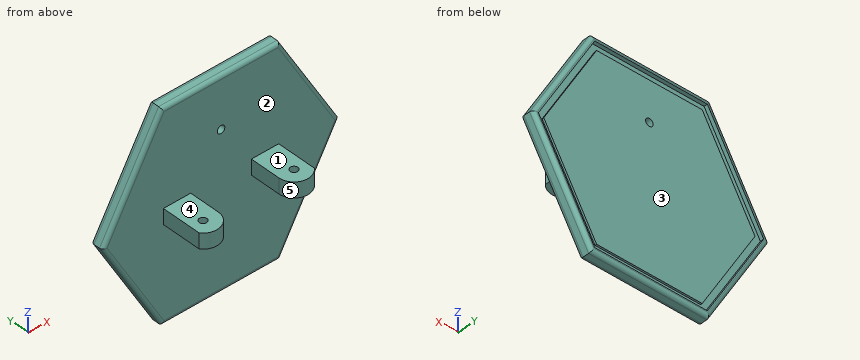
Autodesk Inventor part; units mm, degrees
ref_plane "YZ Plane" through (0, 0, 0) normal (1, 0, 0) x (0, 1, 0)
ref_plane "XZ Plane" through (0, 0, 0) normal (0, 1, 0) x (-1, 0, 0)
ref_plane "XY Plane" through (0, 0, 0) normal (0, 0, 1) x (1, 0, 0)
sketch "스케치1" plane through (0, 0, 0) normal (0, 1, 0) x (-1, 0, 0)
  line L0 (17.6385, -30.5508) -> (-17.6385, -30.5508)
  line L1 (-17.6385, -30.5508) -> (-35.277, 0)
  line L2 (-35.277, 0) -> (-17.6385, 30.5508)
  line L3 (-17.6385, 30.5508) -> (17.6385, 30.5508)
  line L4 (17.6385, 30.5508) -> (35.277, 0)
  line L5 (35.277, 0) -> (17.6385, -30.5508)
  line L6 (19.486, -33.7508) -> (-19.486, -33.7508)
  line L7 (-19.486, -33.7508) -> (-38.972, 0)
  line L8 (-38.972, 0) -> (-19.486, 33.7508)
  line L9 (-19.486, 33.7508) -> (19.486, 33.7508)
  line L10 (19.486, 33.7508) -> (38.972, 0)
  line L11 (38.972, 0) -> (19.486, -33.7508)
  point P0 (0, 0)
  point P1 (0, 0)
  point P2 (0, 0)
  dimension "d0" = 70.554
  dimension "d1" = 3.2
extrude "돌출1" add sketch "스케치1" along normal blind 4.4 contours L0 L1 L2 L3 L4 L5 | L6 L7 L8 L9 L10 L11
sketch "스케치2" plane through (0, 4.4, 0) normal (0, 1, 0) x (1, 0, 0)
  line L0 (-18.5623, 32.1508) -> (18.5623, 32.1508)
  line L1 (18.5623, 32.1508) -> (37.1245, 0)
  line L2 (37.1245, 0) -> (18.5623, -32.1508)
  line L3 (18.5623, -32.1508) -> (-18.5623, -32.1508)
  line L4 (-18.5623, -32.1508) -> (-37.1245, 0)
  line L5 (-37.1245, 0) -> (-18.5623, 32.1508)
  line L6 (-19.486, 33.7508) -> (-38.972, 0)
  point P0 (0, 0)
  point P1 (0, 0)
  dimension "d4" = 1.6
extrude "돌출2" cut sketch "스케치2" against normal blind 1.2
sketch "스케치3" plane through (0, 3.2, 0) normal (0, 1, 0) x (1, 0, 0)
  line L0 (17.4076, -30.1508) -> (-17.4076, -30.1508)
  line L1 (-17.4076, -30.1508) -> (-34.8151, 0)
  line L2 (-34.8151, 0) -> (-17.4076, 30.1508)
  line L3 (-17.4076, 30.1508) -> (17.4076, 30.1508)
  line L4 (17.4076, 30.1508) -> (34.8151, 0)
  line L5 (34.8151, 0) -> (17.4076, -30.1508)
  line L6 (-18.5623, 32.1508) -> (18.5623, 32.1508)
  point P0 (0, 0)
  point P1 (0, 0)
  dimension "d7" = 2
extrude "돌출3" add sketch "스케치3" along normal blind 0.6
fillet "모깎기1" radius 1.2 12 edges at (0, 4.4, -33.7508) (0, 0, -33.7508) (-29.229, 4.4, -16.8754) (-29.229, 0, -16.8754) (-29.229, 4.4, 16.8754) (-29.229, 0, 16.8754) (0, 0, 33.7508) (0, 4.4, 33.7508) (29.229, 0, 16.8754) (29.229, 4.4, 16.8754) (29.229, 4.4, -16.8754) (29.229, 0, -16.8754)
sketch "스케치6" plane through (0, 0, 0) normal (0, -1, 0) x (1, 0, 0)
  line L0 (-20, -2.5) -> (-10, -2.5)
  line L1 (-10, -2.5) -> (-10, 2.5)
  line L2 (-10, 2.5) -> (-20, 2.5)
  line L3 (-20, 2.5) -> (-20, -2.5)
  line L4 (-20, -2.5) -> (-10, 2.5) construction
  line L5 (-10, -2.5) -> (-20, 2.5) construction
  line L6 (10, -2.5) -> (20, -2.5)
  line L7 (20, -2.5) -> (20, 2.5)
  line L8 (20, 2.5) -> (10, 2.5)
  line L9 (10, 2.5) -> (10, -2.5)
  line L10 (10, -2.5) -> (20, 2.5) construction
  line L11 (20, -2.5) -> (10, 2.5) construction
  point P0 (0, 0)
  point P1 (-15, 0)
  point P2 (15, 0)
  point P3 (-10, 0)
  point P4 (10, 0)
  dimension "d27" = 10
  dimension "d28" = 5
  dimension "d29" = 10
  dimension "d30" = 5
  dimension "d31" = 20
  dimension "d32" = 10
extrude "돌출6" add sketch "스케치6" along normal blind 10
sketch "스케치7" plane through (-10, 0, -2.5) normal (0, 0, -1) x (-1, 0, 0)
  line L0 (10, -10) -> (0, -10)
  circle A0 centre (5, -10) radius 5
  line L1 (-30, -10) -> (-20, -10)
  circle A1 centre (-25, -10) radius 5
  point P0 (-10, 0)
extrude "돌출7" add sketch "스케치7" against normal blind 5
sketch "스케치8" plane through (-10, 0, -2.5) normal (0, 0, -1) x (-1, 0, 0)
  arc A0 (0, -10) -> (10, -10) centre (5, -10) ccw
  circle A1 centre (5, -10) radius 1.25
  arc A2 (-30, -10) -> (-20, -10) centre (-25, -10) ccw
  circle A3 centre (-25, -10) radius 1.25
  point P0 (-10, 0)
  dimension "d37" = 2.5
  dimension "d38" = 2.5
extrude "돌출8" cut sketch "스케치8" against normal blind 5
sketch "스케치9" plane through (0, 0, 0) normal (0, -1, 0) x (1, 0, 0)
  line L0 (-20, 2.5) -> (-20, -2.5)
  line L1 (-10, -2.5) -> (-20, -2.5)
  line L2 (-10, -2.5) -> (-10, 2.5)
  line L3 (-20, 2.5) -> (-10, 2.5)
  line L4 (10, 2.5) -> (10, -2.5)
  line L5 (20, -2.5) -> (10, -2.5)
  line L6 (20, -2.5) -> (20, 2.5)
  line L7 (10, 2.5) -> (20, 2.5)
  line L8 (-19, 2.5) -> (-19, -2.5)
  line L9 (19, 2.5) -> (19, -2.5)
  point P0 (0, 0)
  dimension "d41" = 1
  dimension "d42" = 1
extrude "돌출9" cut sketch "스케치9" along normal blind 15 contours L3 L8 L1 L0 | L7 L6 L5 L9
sketch "스케치10" plane through (0, 0, 0) normal (0, -1, 0) x (1, 0, 0)
  circle A0 centre (0, 17) radius 1.25
  point P0 (0, 0)
  dimension "d45" = 2.5
  dimension "d46" = 17
extrude "돌출10" cut sketch "스케치10" against normal up to surface (3.8 mm away)
properties part number "OV-PAM_n_6_bottom"
The listing builds one solid part. Answer for the finished solid, in the listing's coordinates (mm). Face numbers are marked on the shaded views. A direction names the side the tool comes from. Give positions to 0.01 mm unless a question says otherwise; leave off trailing zeros. Write each loop counter-clockwise with the first axis right and the second up, starting at its lowest first coordinate (ties: lowest second). Pieces come first, ordered by that corner, then holes. Notation, with made-up numbers: (25, 89) -> (47, 89) arc R9 ccw to (47, 101) -> close; hole circle Ø10 at (42, 22.5). An arc over 180 degrees is marked (long way). Use one line per item in the form item = value.
1) Each of these flat-tipped pins is pushed along its axis until it touches: P1, Ø2.5, axis at x = -14, y = -8.5, coming from the +Z side; P2, Ø4.5, axis at x = -16.5, y = -4.5, coming from the -Z side; P3, Ø10, axis at y = -1.5, z = -25.5, coming from the +X side; P4, Ø2, axis at x = 15, y = -10, coming from the -Z side. Where does it stop, or does it pass through?
Result:
P1 = 2.5
P2 = -2.5
P3 = 26.74
P4 = through
2) Section A-A on x = 0 is taken. Write down the section's boundary in (y, z), plus the area to 3 significant figures.
Result:
outline = (0, -32.55) arc R1.2 ccw to (1.2, -33.75) -> (3.2, -33.75) arc R1.2 ccw to (4.4, -32.55) -> (4.4, -32.15) -> (3.2, -32.15) -> (3.2, -30.15) -> (3.8, -30.15) -> (3.8, 15.75) -> (0, 15.75) -> close; (0, 18.25) -> (3.8, 18.25) -> (3.8, 30.15) -> (3.2, 30.15) -> (3.2, 32.15) -> (4.4, 32.15) -> (4.4, 32.55) arc R1.2 ccw to (3.2, 33.75) -> (1.2, 33.75) arc R1.2 ccw to (0, 32.55) -> close
area = 245 mm²
3) A tool of negligible diameter and unlimited length cuts with its end or side. For the marked faces 4 and 5, from which of +Z, -Z, +X, -X, +Y, -Y can it reach the whole face along a straight path? Write none if from no direction.
Result:
face_4 = +Z, +X, -X, -Y
face_5 = +Z, -Z, -Y
4) Section C-C on x = 15 is taken. Write down the section's boundary in (y, z).
Result:
outline = (-15, -2.5) -> (-11.25, -2.5) -> (-11.25, 2.5) -> (-15, 2.5) -> close; (-8.75, -2.5) -> (0, -2.5) -> (0, -32.55) arc R1.2 ccw to (1.2, -33.75) -> (3.2, -33.75) arc R1.2 ccw to (4.4, -32.55) -> (4.4, -32.15) -> (3.2, -32.15) -> (3.2, -30.15) -> (3.8, -30.15) -> (3.8, 30.15) -> (3.2, 30.15) -> (3.2, 32.15) -> (4.4, 32.15) -> (4.4, 32.55) arc R1.2 ccw to (3.2, 33.75) -> (1.2, 33.75) arc R1.2 ccw to (0, 32.55) -> (0, 2.5) -> (-8.75, 2.5) -> close
5) For a pull along Z with two mould halves and no side action, classify the marked faces 1, 2 and 3 as +Z half, -Z half, draft (parallel to the pull), parting line (faces both ways), or undercut.
Result:
face_1 = +Z half
face_2 = draft
face_3 = undercut
6) Straight lines are drawn through the part: probe 1 along Y at (x, z) = (15, -1.35); probe 2 along Z at (x, y) = (0, 2.45); probe 3 along Z at (x, y) = (5, 3.5). For each, find the intervals that lie inside material, in ascending order.
Result:
probe_1 = -15 to -11.25, -8.75 to 3.8
probe_2 = -33.75 to 15.75, 18.25 to 33.75
probe_3 = -33.71 to -32.15, -30.15 to 30.15, 32.15 to 33.71
7) Section B-B on y = -1 is taken. Write down the section's boundary in (x, z).
Result:
outline = (-19, -2.5) -> (-10, -2.5) -> (-10, 2.5) -> (-19, 2.5) -> close; (10, -2.5) -> (19, -2.5) -> (19, 2.5) -> (10, 2.5) -> close
